Part model, mm, in its own coordinate system. A direction names the side the tool comes from. Round coordinates to 2 decimals unless told otherwise and drop trailing zeros. Order: outer loops, then holes, each group sorted by start corner. A loop starts at its lowest first (then second) coordinate and runs counter-clockwise, first axis right, second up. Notation, with made-up numbers: (46, -31.5) - (53, -31.5) arc R31 ccw to (53, -4.5) - close; hole circle Ø3 at (17, 46.5). An arc over 180 degrees is marked (long way). Return JSON: item names as keys, results as strings. Group by question number.
Item 1: Saw through at D-D on x = -360.5. List the corners of the cut face in (y, z).
Item 2: Saw through at A-A on y = -48.5. List the corners of the cut face in (x, z), and give its area (3 significant figures).
Item 3: Tool access for faces 1 (the face through (-75, -88, 240)), 2 (the face through (-465, -1, -55)), 3 (the face through (-485, -100, -56)), 4 (the face through (-252.6, -162.32, 224.83)), 5 (the face through (-15, 100, -56)): list every direction of +Z, -Z, +X, -X, +Y, -Y with a clear straight run to the whole face (end or side of a thin tool).
Item 4: Probe probe 1 along Y at (x, z) = (-269, 224.5); probe 2 along Z at (x, y) = (-358, 134.5); probe 3 along Y at (x, z) = (-355, 49). List the from-to ranges inside material, lowest first.
Item 5: Saw through at C-C on z = 205. List the corners of the cut face in (x, y).
Item 6: Saw through at B-B on x = -250. List the corners of the cut face in (y, z).
Item 7: Two-plate mould, pull along Z, no slides. Class faces 6 (the face through (-248, -90, 230)), 7 (the face through (-425, -88, 240)), 8 (the face through (-541, -1, -111.637)), 9 (the face through (-507, -1, -57)): released by +Z, released by -Z, zero draft, split by the parting line, or undercut.
Item 8: Drop flat-ended pins along their axis: pin 1 (10 mm diameter, centred on y = -84.5, z = 243.5, fed in from +X); pin 2 (6 mm diameter, centred on x = -30.5, y = 28.5, fed in from -Z); pin 3 (2 mm diameter, centred on y = -131.5, z = 136.5, fed in from -X). Give the stop position or say it passes through.
```python
from build123d import *

# Parameters (mm, degrees)
F1_DEPTH  = 150
F3_DEPTH  = 100
F7_DEPTH  = 1
F8_R      = 20
F9_DEPTH  = 25
F11_DEPTH = 175


with BuildPart() as f1:
    # F0 (on Front) → F1 (new body, symmetric)
    with BuildSketch(Plane.XZ):
        with BuildLine():
            Line((-500, 0), (0, 0))
            ThreePointArc((0, 0), (125, 125), (0, 250))
            Line((0, 250), (-500, 250))
            ThreePointArc((-500, 250), (-625, 125), (-500, 0))
        make_face()
    extrude(amount=F1_DEPTH, both=True)

    # F2 (on Front) → F3 (join, symmetric)
    with BuildSketch(Plane.XZ):
        Polygon((61.636794, -111.636794), (-50, 0), (-90, 0), (21.636792, -111.636794), align=None)
    extrude(amount=F3_DEPTH, both=True)

    # F5: F1 across plane


with BuildPart() as f1_1:
    add(f1.part)
    add(f1.part.mirror(Plane.YZ.offset(-250)))

    # F6 (on face) → F7 (join)
    with BuildSketch(Plane.XZ.offset(150)):
        with BuildLine():
            ThreePointArc((-500, 25), (-429.289322, 54.289322), (-400, 125))
            ThreePointArc((-400, 125), (-405.13167, 156.622777), (-420, 185))
            ThreePointArc((-420, 185), (-589.442719, 169.72136), (-500, 25))
        make_face()
        with BuildLine():
            ThreePointArc((-420, 185), (-405.13167, 156.622777), (-400, 125))
            ThreePointArc((-400, 125), (-429.289322, 54.289322), (-500, 25))
            Line((-500, 25), (0, 25))
            ThreePointArc((0, 25), (-89.442719, 80.27864), (-80, 185))
            ThreePointArc((-80, 185), (-250, 105), (-420, 185))
        make_face()
        with BuildLine():
            ThreePointArc((100, 125), (31.622777, 219.86833), (-80, 185))
            ThreePointArc((-80, 185), (-89.442719, 80.27864), (0, 25))
            ThreePointArc((0, 25), (70.710678, 54.289322), (100, 125))
        make_face()
    extrude(amount=F7_DEPTH)

    # F8 (on face) → F9 (join)
    with BuildSketch(Plane.XZ.offset(150)):
        with Locations((-250, 205)):
            Circle(F8_R)
    extrude(amount=F9_DEPTH)

    # F10 (on offset) → F11 (cut, symmetric)
    with BuildSketch(Plane.YZ.offset(-250)):
        Polygon((-68, 250.78461), (-100, 250.78461), (-100, 230), (-80, 230), align=None)
    extrude(amount=F11_DEPTH, both=True, mode=Mode.SUBTRACT)


solid = f1_1.part
```
Filled in:
{
 "1": {"outline": "(-151, 25) - (-150, 25) - (-150, 0) - (150, 0) - (150, 250) - (-68.45, 250) - (-80, 230) - (-100, 230) - (-100, 250) - (-150, 250) - (-150, 134.67) - (-151, 134.67) - close"},
 "2": {"outline": "(-561.64, -111.64) - (-521.64, -111.64) - (-410, 0) - (-90, 0) - (21.64, -111.64) - (61.64, -111.64) - (-50, 0) - (0, 0) arc R125 ccw to (0, 250) - (-500, 250) arc R125 ccw to (-500, 0) - (-450, 0) - close", "area": "183,000 mm^2"},
 "3": {"face 1": "+Z", "face 2": "-Z, +Y, -Y", "face 3": "-Z, +X, -X, -Y", "face 4": "-Y", "face 5": "-Z, +X, -X, +Y"},
 "4": {"probe 1": "y = -150 to 150", "probe 2": "z = 0 to 250", "probe 3": "y = -151 to 150"},
 "5": {"outline": "(-596.05, -150) - (-560, -150) - (-560, -151) - (-440, -151) - (-440, -150) - (-270, -150) - (-270, -175) - (-230, -175) - (-230, -150) - (-60, -150) - (-60, -151) - (60, -151) - (60, -150) - (96.05, -150) - (96.05, 150) - (-596.05, 150) - close"},
 "6": {"outline": "(-175, 185) - (-150, 185) - (-150, 105) - (-151, 105) - (-151, 25) - (-150, 25) - (-150, 0) - (150, 0) - (150, 250) - (-68.45, 250) - (-80, 230) - (-100, 230) - (-100, 250) - (-150, 250) - (-150, 225) - (-175, 225) - close"},
 "7": {"face 6": "released by +Z", "face 7": "zero draft", "face 8": "released by -Z", "face 9": "undercut"},
 "8": {"pin 1": "stops at x = 52.37", "pin 2": "stops at z = -62.5", "pin 3": "stops at x = -624.56"}
}
